Check sheet for the modelled part. Datum: model origin and axes. Units: mm. A direction names the side the tool comes from. Round coordinates to 2 decimals unless told otherwise and drop trailing zeros. Order: outer loops, then holes, each group sorted by start corner. A loop starts at its lowest first (then second) coordinate and runs counter-clockwise, first axis right, second up.
from build123d import *
from OCP.BRepFilletAPI import BRepFilletAPI_MakeChamfer

# Parameters (mm, degrees)
SKETCH1_W           = 43
SKETCH1_H           = 43
SKETCH1_R           = 11
BOSS_EXTRUDE1_DEPTH = 20.67
SKETCH2_R           = 12.5
CUT_EXTRUDE1_DEPTH  = 3
SKETCH3_R           = 1.5
CUT_EXTRUDE2_DEPTH  = 37.766137953
SKETCH4_W           = 23
SKETCH4_H           = 12.67
CUT_EXTRUDE3_DEPTH  = 20
SKETCH5_R           = 3
CUT_EXTRUDE4_DEPTH  = 3
FILLET1_R           = 2
CHAMFER1_SIZE       = 1
CHAMFER1_SIZE2      = 0.600860619


with BuildPart() as part:
    # Sketch1 → Boss-Extrude1 (new body)
    with BuildSketch(Plane(origin=(0, 0, 0), x_dir=(1, 0, 0), z_dir=(0, 1, 0))):
        Rectangle(SKETCH1_W, SKETCH1_H)
        with Locations(Location((0, 0, 0), (0, 0, 270))):
            Circle(SKETCH1_R, mode=Mode.SUBTRACT)
    extrude(amount=BOSS_EXTRUDE1_DEPTH)

    # Sketch2 → Cut-Extrude1 (cut)
    with BuildSketch(Plane.XZ):
        with Locations(Location((0, 0, 0), (0, 0, 270))):
            Circle(SKETCH2_R)
    extrude(amount=-CUT_EXTRUDE1_DEPTH, mode=Mode.SUBTRACT)

    # Sketch3 → Cut-Extrude2 (cut, through all)
    with BuildSketch(Plane(origin=(0, 20.67, 0), x_dir=(1, 0, 0), z_dir=(0, 1, 0))):
        with Locations(Location((-15.5, 15.5, 0), (0, 0, 270))):
            Circle(SKETCH3_R)
        with Locations(Location((15.5, 15.5, 0), (0, 0, 270))):
            Circle(SKETCH3_R)
        with Locations(Location((15.5, -15.5, 0), (0, 0, 270))):
            Circle(SKETCH3_R)
        with Locations(Location((-15.5, -15.5, 0), (0, 0, 270))):
            Circle(SKETCH3_R)
    extrude(amount=-CUT_EXTRUDE2_DEPTH, mode=Mode.SUBTRACT)

    # Sketch4 → Cut-Extrude3 (cut)
    with BuildSketch(Plane.XY.offset(21.5)):
        with Locations((0, 10.335)):
            Rectangle(SKETCH4_W, SKETCH4_H)
    extrude(amount=-CUT_EXTRUDE3_DEPTH, mode=Mode.SUBTRACT)

    # Sketch5 → Cut-Extrude4 (cut)
    with BuildSketch(Plane(origin=(0, 20.67, 0), x_dir=(1, 0, 0), z_dir=(0, 1, 0))):
        with Locations(Location((-15.5, 15.5, 0), (0, 0, 270))):
            Circle(SKETCH5_R)
        with Locations(Location((15.5, 15.5, 0), (0, 0, 270))):
            Circle(SKETCH5_R)
        with Locations(Location((15.5, -15.5, 0), (0, 0, 270))):
            Circle(SKETCH5_R)
        with Locations(Location((-15.5, -15.5, 0), (0, 0, 270))):
            Circle(SKETCH5_R)
    extrude(amount=-CUT_EXTRUDE4_DEPTH, mode=Mode.SUBTRACT)

    # Fillet1
    fillet1_edges = [part.edges().sort_by_distance(p)[0] for p in [
        (21.5, 10.335, 21.5),
        (-21.5, 10.335, 21.5),
        (-21.5, 10.335, -21.5),
        (21.5, 10.335, -21.5),
    ]]
    fillet(fillet1_edges, radius=FILLET1_R)

    # Chamfer1: one chamfer whose edges measure the first distance from different faces: ONE call of the kernel's chamfer builder (chamfer() names one face for all edges)
    chamfer1_edges_1 = [part.edges().sort_by_distance(p)[0] for p in [
        (11.5, 10.335, 1.5),
    ]]
    chamfer1_side_1 = [part.faces().sort_by_distance(p)[0] for p in [
        (11.5, 10.335, 11.5),
    ]]
    chamfer1_edges_2 = [part.edges().sort_by_distance(p)[0] for p in [
        (-11.5, 10.335, 1.5),
    ]]
    chamfer1_side_2 = [part.faces().sort_by_distance(p)[0] for p in [
        (-11.5, 10.335, 11.5),
    ]]
    chamfer1 = BRepFilletAPI_MakeChamfer(part.part.solid().wrapped)
    for e in chamfer1_edges_1:
        chamfer1.Add(CHAMFER1_SIZE, CHAMFER1_SIZE2, e.wrapped, chamfer1_side_1[0].wrapped)  # the first distance lies on this face
    for e in chamfer1_edges_2:
        chamfer1.Add(CHAMFER1_SIZE, CHAMFER1_SIZE2, e.wrapped, chamfer1_side_2[0].wrapped)  # the first distance lies on this face
    add(Compound.cast(chamfer1.Shape()), mode=Mode.REPLACE)


solid = part.part
1) Scan lines: line 1 (X direction, y = 19.6, z = -15.5); line 2 (X direction, y = 5, z = 15.5); line 3 (X direction, y = 13.5, z = -15.5). Record each from-to range of solid material in increasing order.
2) Gauge pin test, flat ends, axial feed: pin 1 (6 mm diameter, centred on x = -2, y = 10.5, fed in from +Z); pin 2 (1.8 mm diameter, centred on x = 16.5, z = 14.5, fed in from +Y). Record the tip position at first contact, or that the pin passes through.
3) Draft check along X on faces 1 (the face through (-17, 17.67, 17)), 2 (the face through (-20.93, 10.48, -20.9)), 3 (the face through (9, 0, 9)). Enter one of: pulls with the +X half, pulls with the -X half, needs draft (parallel to the pull), parting line crosses it, or undercut.
4) Sectioned sample at D-D on y = 13.25. Count the separate pieces of the cut face and the enclosed holes in it, and give its area (3 significant figures).
5) Set-up check for faces 4 (the face through (3.755, 1.479, -11.923)), 5 (the face through (14, 17.67, 17)), 6 (the face through (15.57, 8.96, 14)), 7 (the face through (0, 16.67, 14)): record each of +Z, -Z, +X, -X, +Y, -Y from which the full face is reachable in a straight line by a thin tool's end or side.
6) Sectioned sample at C-C on y = 2.25. Record the cut outline in (x, z).
7) Sectioned sample at B-B on x = -15.5. Record the cut outline in (y, z).
8) Sectioned sample at A-A on z = 15.5. Record the cut outline in (x, y).
Values found:
1. line 1: x = -21.5 to -18.5, -12.5 to 12.5, 18.5 to 21.5
1. line 2: x = -21.5 to -17, -14 to -11.5, 11.5 to 14, 17 to 21.5
1. line 3: x = -21.5 to -17, -14 to 14, 17 to 21.5
2. pin 1: stops at z = -9.8
2. pin 2: stops at y = 17.67
3. face 1: undercut
3. face 2: pulls with the -X half
3. face 3: needs draft
4. separate pieces: 1
4. enclosed holes: 4
4. area: 1,130 mm2
5. face 4: -Y
5. face 5: +Y
5. face 6: +Y, -Y
5. face 7: +Z
6. outline: (-21.5, -19.5) arc R2 ccw to (-19.5, -21.5) - (19.5, -21.5) arc R2 ccw to (21.5, -19.5) - (21.5, 19.5) arc R2 ccw to (19.5, 21.5) - (-19.5, 21.5) arc R2 ccw to (-21.5, 19.5) - close; hole circle Ø3 at (-15.5, -15.5); hole circle Ø3 at (-15.5, 15.5); hole circle Ø25 at (0, 0); hole circle Ø3 at (15.5, -15.5); hole circle Ø3 at (15.5, 15.5)
7. outline: (0, -21.5) - (20.67, -21.5) - (20.67, -18.5) - (17.67, -18.5) - (17.67, -17) - (0, -17) - close; (0, -14) - (17.67, -14) - (17.67, -12.5) - (20.67, -12.5) - (20.67, 12.5) - (17.67, 12.5) - (17.67, 14) - (0, 14) - close; (0, 17) - (17.67, 17) - (17.67, 18.5) - (20.67, 18.5) - (20.67, 21.5) - (0, 21.5) - close
8. outline: (-21.5, 0) - (-17, 0) - (-17, 17.67) - (-18.5, 17.67) - (-18.5, 20.67) - (-21.5, 20.67) - close; (-14, 0) - (14, 0) - (14, 17.67) - (12.5, 17.67) - (12.5, 20.67) - (-12.5, 20.67) - (-12.5, 17.67) - (-14, 17.67) - close; (17, 0) - (21.5, 0) - (21.5, 20.67) - (18.5, 20.67) - (18.5, 17.67) - (17, 17.67) - close; hole (-11.5, 4) - (11.5, 4) - (11.5, 16.67) - (-11.5, 16.67) - close
